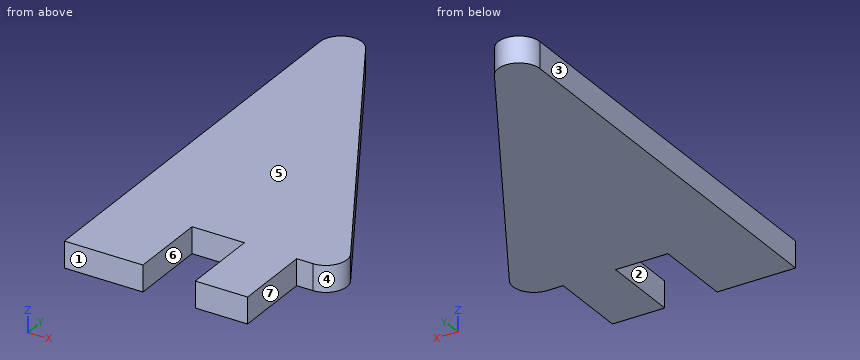
from build123d import *

# Parameters (mm, degrees)
SKETCH1_W           = 9.525
SKETCH1_H           = 9.525
SKETCH1_W_2         = 6.35
BOSS_EXTRUDE1_DEPTH = 3.175
FILLET1_R           = 2.54


with BuildPart() as part:
    # Sketch1 → Boss-Extrude1 (new body)
    with BuildSketch(Plane.XY):
        Polygon((28.575, 0), (0, 0), (0, 49.493351826), align=None)
        with Locations((4.7625, -4.7625)):
            Rectangle(SKETCH1_W, SKETCH1_H)
        with Locations((19.05, -4.7625)):
            Rectangle(SKETCH1_W_2, SKETCH1_H)
    extrude(amount=BOSS_EXTRUDE1_DEPTH)

    # Fillet1
    fillet1_edges = [part.edges().sort_by_distance(p)[0] for p in [
        (0, 49.493351826, 1.5875),
        (28.575, 0, 1.5875),
    ]]
    fillet(fillet1_edges, radius=FILLET1_R)


solid = part.part
Here's how the part is built. I have some questions about the finished solid (model axes, mm). Face numbers are marked on the shaded views. A direction names the side the tool comes from. Coordinates: 2 decimals unless noted, no trailing zeros. Write each loop counter-clockwise with the first axis right and the second up, starting at its lowest first coordinate (ties: lowest second). Pieces come first, ordered by that corner, then holes.
1) If we section it at B-B (y = 4.5): List the corners of the cut face in (x, z) for me (3 decimals).
Filled in:
outline: (0, 0) - (25.977, 0) - (25.977, 3.175) - (0, 3.175) - close
2) Which directions (+Z, -Z, +X, -X, +Y, -Y) give clear straight access to the entire face, cutting with the end or side of a thin tool? Please do the marked faces 5, 6 and 7.
Filled in:
face 5: +Z, +X, -X, +Y, -Y
face 6: +Z, -Z, -Y
face 7: +Z, -Z, +X, -Y
3) I'm going to push flat-ended pins straight in: pin 1 (12 mm diameter, centred on x = 8, y = 30.5, fed in from -Z); pin 2 (1 mm diameter, centred on x = 15, z = 2.5, fed in from -Y); pin 3 (1 mm diameter, centred on x = 16.5, z = 2.5, fed in from +Y); pin 4 (1 mm diameter, centred on y = -3.5, z = 1.5, fed in from +X) (3 decimals). Where does each tip first touch, or does it pass through?
Filled in:
pin 1: stops at z = 0
pin 2: stops at y = 0
pin 3: stops at y = 21.78
pin 4: stops at x = 22.225
4) If we section it at C-C (x = 22.75): List the corners of the cut face in (y, z) for me (3 decimals).
Filled in:
outline: (0, 0) - (10.089, 0) - (10.089, 3.175) - (0, 3.175) - close
5) If we section it at A-A (z = 2.4): List the corners of the cut face in (x, y) for me (3 decimals).
Filled in:
outline: (0, -9.525) - (9.525, -9.525) - (9.525, 0) - (15.875, 0) - (15.875, -9.525) - (22.225, -9.525) - (22.225, 0) - (24.176, 0) arc R2.54 ccw to (26.375, 3.81) - (4.74, 41.284) arc R2.54 ccw to (0, 40.014) - close
6) Thinking about a two-plate mould opening in X: for the marked faces 1, 2, 3 and 4, which applies, +X half, -X half, draft (parallel to the pull), parting line (faces both ways), or undercut?
Filled in:
face 1: draft
face 2: undercut
face 3: -X half
face 4: +X half
7) If I drill on line 1 (X direction, y = -4.5, z = 2.9) (3 decimals); line 2 (X direction, y = 11, z = 1.9); line 3 (Y direction, x = 23.25, z = 2.95), over which ranges is the centre line in solid material (lowest first)?
Filled in:
line 1: x = 0 to 9.525, 15.875 to 22.225
line 2: x = 0 to 22.22
line 3: y = 0 to 9.22
